Check sheet for the modelled part. Datum: model origin and axes. Units: mm. A direction names the side the tool comes from. Coordinates: 2 decimals unless noted, no trailing zeros. Loops run counter-clockwise (first coordinate to the right, second up) from the corner with the lowest first, then second, coordinate; pieces in that order, holes last. Notation, with made-up numbers: M 79.25,14.5 L 136.25,14.5 A12 ccw 136.25,21.5 Z; hole C 15.5,12 d9. An arc over 180 degrees is marked long. Write each question's results on one line, items separated by ' | '. Start each with the question number.
from build123d import *

# Parameters (mm, degrees)
SKETCH1_W           = 50.8
SKETCH1_H           = 38.1
BOSS_EXTRUDE1_DEPTH = 20.32
SKETCH2_R           = 2.54
BOSS_EXTRUDE2_DEPTH = 27.94


with BuildPart() as part:
    # Sketch1 → Boss-Extrude1 (new body)
    with BuildSketch(Plane(origin=(0, 0, 0), x_dir=(1, 0, 0), z_dir=(0, 1, 0))):
        Rectangle(SKETCH1_W, SKETCH1_H)
    extrude(amount=BOSS_EXTRUDE1_DEPTH)

    # Sketch2 → Boss-Extrude2 (add)
    with BuildSketch(Plane(origin=(0, 20.32, 0), x_dir=(1, 0, 0), z_dir=(0, 1, 0))):
        with Locations(Location((-20.32, 13.97, 0), (0, 0, 90))):
            Circle(SKETCH2_R)
        with Locations(Location((-20.32, -13.97, 0), (0, 0, 90))):
            Circle(SKETCH2_R)
        with Locations(Location((-20.32, 0, 0), (0, 0, 90))):
            Circle(SKETCH2_R)
    extrude(amount=BOSS_EXTRUDE2_DEPTH)


solid = part.part
1) Section check D-D (x = -7). Enter the section's corners in (y, z), then the cut area to 3 significant figures.
2) Gauge pin test, flat ends, axial feed: P1, Ø19, axis at x = 7.5, z = 8.5, coming from the +Y side; P2, Ø8, axis at x = -14, y = 26.5, coming from the +Z side. Record the tip position at first contact, or that the pin passes through.
3) Set-up check for faces 4 (the cylindrical face through (-20.432, 34.094, 16.508)), 5 (the flat face through (-25.4, 10, 0)): record each of +Z, -Z, +X, -X, +Y, -Y from which the full face is reachable in a straight line by a thin tool's end or side.
4) Section check A-A (y = 27.5). Enter the section's corners in (x, z), then the cut area to 3 significant figures.
5) Thickness scan on probe 1 along Z at (x, y) = (-20.5, 25); probe 2 along Z at (x, y) = (-20, 28.5); probe 3 along Y at (x, z) = (12, 5). Record the ranges inside material, lowest first.
6) Section check B-B (x = -20.32). Enter the section's corners in (y, z), then the cut area to 3 significant figures.
7) Section check C-C (z = 13.97). Enter the section's corners in (x, y), then the cut area to 3 significant figures.
8) Release check for a two-part mould opening along Z. For faces 1 (the cylindrical face through (-18.067, 34.094, -1.172)), 2 (the flat face through (-20, 48.26, 0)), 3 (the flat face through (0, 10, 19.05)) record: +Z half, -Z half, draft (parallel to the pull), parting line (faces both ways), or undercut.
Return value:
1) outline: M 0,-19.05 L 20.32,-19.05 L 20.32,19.05 L 0,19.05 Z | area: 774 mm2
2) P1: stops at y = 20.32 | P2: stops at z = 15
3) face 4: +Y | face 5: +Z, -Z, -X, +Y, -Y
4) outline: C -20.32,-13.97 d5.08; C -20.32,0 d5.08; C -20.32,13.97 d5.08 | area: 60.8 mm2
5) probe 1: z = -16.5 to -11.44, -2.53 to 2.53, 11.44 to 16.5 | probe 2: z = -16.49 to -11.45, -2.52 to 2.52, 11.45 to 16.49 | probe 3: y = 0 to 20.32
6) outline: M 0,-19.05 L 20.32,-19.05 L 20.32,-16.51 L 48.26,-16.51 L 48.26,-11.43 L 20.32,-11.43 L 20.32,-2.54 L 48.26,-2.54 L 48.26,2.54 L 20.32,2.54 L 20.32,11.43 L 48.26,11.43 L 48.26,16.51 L 20.32,16.51 L 20.32,19.05 L 0,19.05 Z | area: 1,200 mm2
7) outline: M -25.4,0 L 25.4,0 L 25.4,20.32 L -17.78,20.32 L -17.78,48.26 L -22.86,48.26 L -22.86,20.32 L -25.4,20.32 Z | area: 1,170 mm2
8) face 1: undercut | face 2: draft | face 3: +Z half
